Can you work these out from the model? Positions are in its coordinate system, mm. A direction names the side the tool comes from. Coordinates: 2 decimals unless noted, no trailing zeros. Loops run counter-clockwise (first coordinate to the right, second up) from the corner with the lowest first, then second, coordinate; pieces in that order, holes last. Notation, with made-up numbers: M -1.5,25 L 49.5,25 A31 ccw 49.5,51 Z; hole C 60.5,43.5 d10. An arc over 180 degrees is marked long. Answer as a JSON object with one key per item and string values. Group by question number.
Item 1: Which directions (+Z, -Z, +X, -X, +Y, -Y) give clear straight access to the entire face, cutting with the end or side of a thin tool? Please do faces 1 (the cylindrical face through (-21.64, 29.1, 1.62)), 2 (the flat face through (-13, -21, 1.6)).
Item 2: Suppose I cut it at D-D (z = 0.85). Count the separate pieces of the cut face and the enclosed holes in it, then the cut area to 3 significant figures.
Item 3: Suppose I cut it at A-A (y = 20). Write out the boundary of the cut face in (x, z), then the cut area to 3 significant figures.
Item 4: I'm going to push a flat-ended pin straight in: pin 1 Ø5.5 at (x, y) = (11.43, 20) entering from -Z. Where does the tip first touch, or does it pass through?
Item 5: Suppose I cut it at C-C (y = 0). Write out the boundary of the cut face in (x, z).
Item 6: If I drill on line 1 (Y direction, x = 11.43, z = 2); line 2 (Y direction, x = 19.5, z = 0.85); line 3 (X direction, y = -20, z = 2.4), over which ranges is the centre line in solid material (lowest first)?
Item 7: Suppose I cut it at B-B (x = -11.43). Write out the boundary of the cut face in (y, z).
```python
from build123d import *

# Parameters (mm, degrees)
SKETCH_1_W          = 45
SKETCH_1_H          = 60
EXTRUDE_1_DEPTH     = 3.2
SKETCH_3_R          = 1.7
CUT_EXTRUDE_2_DEPTH = 38.636285683
SKETCH_2_R          = 1.7
CUT_EXTRUDE_1_DEPTH = 38.636285683
FILLET_1_R          = 3
SKETCH_4_R          = 3
CUT_EXTRUDE_3_DEPTH = 1.6


with BuildPart() as part:
    # 草圖1 → 填料-伸長1 (new body)
    with BuildSketch(Plane.XY):
        Rectangle(SKETCH_1_W, SKETCH_1_H)
    extrude(amount=EXTRUDE_1_DEPTH)

    # 草圖3 → 除料-伸長2 (cut, through all)
    with BuildSketch(Plane.XY.offset(3.2)):
        with Locations((-11.43, 0)):
            Circle(SKETCH_3_R)
        with Locations((11.43, 0)):
            Circle(SKETCH_3_R)
        with Locations((11.43, 20)):
            Circle(SKETCH_3_R)
        with Locations((-11.43, 20)):
            Circle(SKETCH_3_R)
        with Locations(Location((-11.43, -20, 0), (0, 0, 180))):
            Circle(SKETCH_3_R)
        with Locations(Location((11.43, -20, 0), (0, 0, 180))):
            Circle(SKETCH_3_R)
    extrude(amount=-CUT_EXTRUDE_2_DEPTH, mode=Mode.SUBTRACT)

    # 草圖2 → 除料-伸長1 (cut, through all)
    with BuildSketch(Plane.XY.offset(3.2)):
        with Locations((-19.5, 20)):
            Circle(SKETCH_2_R)
        with Locations((19.5, 20)):
            Circle(SKETCH_2_R)
        with Locations(Location((19.5, -20, 0), (0, 0, 180))):
            Circle(SKETCH_2_R)
        with Locations(Location((-19.5, -20, 0), (0, 0, 180))):
            Circle(SKETCH_2_R)
    extrude(amount=-CUT_EXTRUDE_1_DEPTH, mode=Mode.SUBTRACT)

    # 圓角1
    fillet_1_edges = [part.edges().sort_by_distance(p)[0] for p in [
        (-22.5, 30, 1.6),
        (22.5, 30, 1.6),
        (22.5, -30, 1.6),
        (-22.5, -30, 1.6),
    ]]
    fillet(fillet_1_edges, radius=FILLET_1_R)

    # 草圖4 → 除料-伸長3 (cut)
    with BuildSketch(Plane(origin=(0, 0, 0), x_dir=(-1, 0, 0), z_dir=(0, 0, -1))):
        with Locations((-11.43, 20)):
            Circle(SKETCH_4_R)
        with Locations((11.43, 20)):
            Circle(SKETCH_4_R)
        with Locations((-11.43, 0)):
            Circle(SKETCH_4_R)
        with Locations((11.43, 0)):
            Circle(SKETCH_4_R)
        with Locations((-11.43, -20)):
            Circle(SKETCH_4_R)
        with Locations((11.43, -20)):
            Circle(SKETCH_4_R)
    extrude(amount=-CUT_EXTRUDE_3_DEPTH, mode=Mode.SUBTRACT)


solid = part.part
```
From the geometry:
{
 "1": {"face 1": "+Z, -Z, -X, +Y", "face 2": "-Z"},
 "2": {"separate pieces": "1", "enclosed holes": "10", "area": "2,490 mm2"},
 "3": {"outline": "M -22.5,0 L -21.2,0 L -21.2,3.2 L -22.5,3.2 Z; M -17.8,0 L -14.43,0 L -14.43,1.6 L -13.13,1.6 L -13.13,3.2 L -17.8,3.2 Z; M -9.73,1.6 L -8.43,1.6 L -8.43,0 L 8.43,0 L 8.43,1.6 L 9.73,1.6 L 9.73,3.2 L -9.73,3.2 Z; M 13.13,1.6 L 14.43,1.6 L 14.43,0 L 17.8,0 L 17.8,3.2 L 13.13,3.2 Z; M 21.2,0 L 22.5,0 L 22.5,3.2 L 21.2,3.2 Z", "area": "92.2 mm2"},
 "4": {"pin 1": "z = 1.6"},
 "5": {"outline": "M -22.5,0 L -14.43,0 L -14.43,1.6 L -13.13,1.6 L -13.13,3.2 L -22.5,3.2 Z; M -9.73,1.6 L -8.43,1.6 L -8.43,0 L 8.43,0 L 8.43,1.6 L 9.73,1.6 L 9.73,3.2 L -9.73,3.2 Z; M 13.13,1.6 L 14.43,1.6 L 14.43,0 L 22.5,0 L 22.5,3.2 L 13.13,3.2 Z"},
 "6": {"line 1": "-30 to -21.7, -18.3 to -1.7, 1.7 to 18.3, 21.7 to 30", "line 2": "-30 to -21.7, -18.3 to 18.3, 21.7 to 30", "line 3": "-22.5 to -21.2, -17.8 to -13.13, -9.73 to 9.73, 13.13 to 17.8, 21.2 to 22.5"},
 "7": {"outline": "M -30,0 L -23,0 L -23,1.6 L -21.7,1.6 L -21.7,3.2 L -30,3.2 Z; M -18.3,1.6 L -17,1.6 L -17,0 L -3,0 L -3,1.6 L -1.7,1.6 L -1.7,3.2 L -18.3,3.2 Z; M 1.7,1.6 L 3,1.6 L 3,0 L 17,0 L 17,1.6 L 18.3,1.6 L 18.3,3.2 L 1.7,3.2 Z; M 21.7,1.6 L 23,1.6 L 23,0 L 30,0 L 30,3.2 L 21.7,3.2 Z"}
}
